Design review of the part built by this model. Coordinates are the model's own, in mm. Face numbers are marked on the shaded views. Coordinates: 2 decimals unless noted, no trailing zeros. Write each loop counter-clockwise with the first axis right and the second up, starting at its lowest first coordinate (ties: lowest second). Pieces come first, ordered by that corner, then holes. Notation, with made-up numbers: (-19, 73.25) -> (10, 73.25) arc R13 ccw to (10, 78.25) -> close; hole circle Ø8 at (65, 65.5). An arc over 180 degrees is marked (long way). Answer in a Markdown table with one row per item. Add a question column.
Item 1: Take a section at A-A, the plane z = 32. Write out the cut boundary in (x, y), and give its area (3 significant figures).
Item 2: To check wall thickness, follow line 1 (X direction, y = 1.35, z = 48); line 2 (X direction, y = 5.5, z = 21.5); line 3 (Y direction, x = -42, z = -11). State the ranges of each line that lie inside material, in increasing order.
Item 3: Take a section at B-B, the plane z = -20. Write out the cut boundary in (x, y).
Item 4: Clearance check with flat-ended pins moving along their axes: P1, Ø1.5, axis at y = 9, z = -24, coming from the +X side; P2, Ø6.5, axis at x = 43.5, z = -16, coming from the +Y side; P3, Ø6, axis at y = 12, z = -2, coming from the -X side. State where each tip first meets the part, or that it passes through.
Item 5: Draft analysis for pull direction X (two halves, no side actions). For the marked faces 1, 2 and 3, state which applies: released by +X, released by -X, zero draft, split by the parting line, or undercut.
Item 6: Take a section at C-C, the plane y = 16.25. Write out the cut boundary in (x, z), and give its area (3 significant figures).
Autodesk Inventor part; units mm, degrees
ref_plane "YZ Plane" through (0, 0, 0) normal (1, 0, 0) x (0, 1, 0)
ref_plane "XZ Plane" through (0, 0, 0) normal (0, 1, 0) x (-1, 0, 0)
ref_plane "XY Plane" through (0, 0, 0) normal (0, 0, 1) x (1, 0, 0)
sketch "Sketch1" plane through (0, 0, 0) normal (0, 1, 0) x (-1, 0, 0)
  line L0 (-47.5, -52) -> (47.5, -52)
  line L1 (47.5, -52) -> (47.5, 52)
  line L2 (47.5, 52) -> (-47.5, 52)
  line L3 (-47.5, 52) -> (-47.5, -52)
  line L4 (-47.5, -52) -> (47.5, 52) construction
  line L5 (47.5, -52) -> (-47.5, 52) construction
  point P0 (0, 0)
  dimension "d0" = 95
  dimension "d1" = 104
extrude "Extrusion1" add sketch "Sketch1" along normal blind 3
sketch "Sketch2" plane through (0, 3, 0) normal (0, 1, 0) x (1, 0, 0)
  line L0 (-47.5, -52) -> (47.5, -52)
  line L1 (37.5, 52) -> (-37.5, 52)
  line L2 (-37.5, 52) -> (-37.5, -52)
  line L3 (-37.5, -52) -> (37.5, -52)
  line L4 (37.5, -52) -> (37.5, 52)
  line L5 (37.5, 52) -> (-37.5, -52) construction
  line L6 (-37.5, 52) -> (37.5, -52) construction
  point P0 (0, 0)
  dimension "d4" = 75
  dimension "d5" = 104
extrude "Extrusion2" add sketch "Sketch2" along normal blind 20
sketch "Sketch3" plane through (0, 0, 0) normal (0, -1, 0) x (1, 0, 0)
  line L0 (-47.5, 52) -> (-43.5, 52)
  line L1 (-43.5, 52) -> (-43.5, 48)
  line L2 (-43.5, 48) -> (-47.5, 48)
  line L3 (-47.5, 48) -> (-47.5, 52)
  line L4 (-47.5, 52) -> (47.5, 52)
  line L5 (47.5, 52) -> (43.5, 52)
  line L6 (43.5, 52) -> (43.5, 48)
  line L7 (43.5, 48) -> (47.5, 48)
  line L8 (47.5, 48) -> (47.5, 52)
  circle A0 centre (-43.5, 48) radius 1.85
  circle A1 centre (-43.5, 32) radius 1.85
  circle A2 centre (-43.5, 16) radius 1.85
  circle A3 centre (-43.5, 0) radius 1.85
  circle A4 centre (-43.5, -16) radius 1.85
  circle A5 centre (-43.5, -32) radius 1.85
  circle A6 centre (-43.5, -48) radius 1.85
  circle A7 centre (43.5, -48) radius 1.85
  circle A8 centre (43.5, -32) radius 1.85
  circle A9 centre (43.5, -16) radius 1.85
  circle A10 centre (43.5, 0) radius 1.85
  circle A11 centre (43.5, 16) radius 1.85
  circle A12 centre (43.5, 32) radius 1.85
  circle A13 centre (43.5, 48) radius 1.85
  point P0 (0, 0)
  dimension "d8" = 4
  dimension "d9" = 4
  dimension "d10" = 4
  dimension "d11" = 4
hole "Hole2" at (-43.5, 0, 48) at (-43.5, 0, 32) at (-43.5, 0, 16) at (-43.5, 0, 0) at (-43.5, 0, -16) at (-43.5, 0, -32) at (-43.5, 0, -48) at (43.5, 0, -48) at (43.5, 0, -32) at (43.5, 0, -16) at (43.5, 0, 0) at (43.5, 0, 16) at (43.5, 0, 32) at (43.5, 0, 48) direction (0, 1, 0) diameter 4 end through all
properties part number "CPD Module"
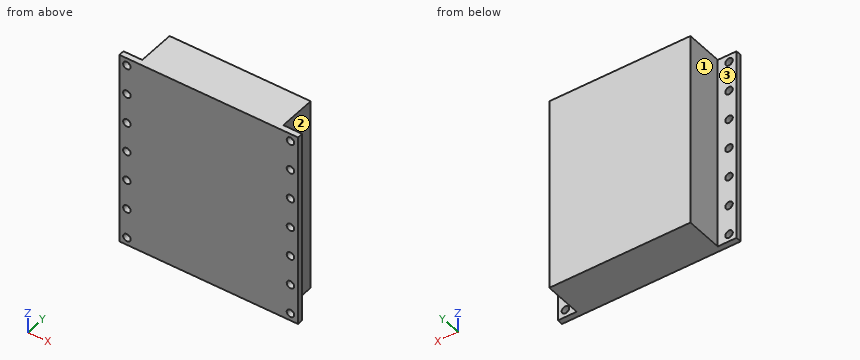
Answers:
| question | item | result |
|---|---|---|
| 1 | outline | (-47.5, 0) -> (-45.5, 0) -> (-45.5, 3) -> (-47.5, 3) -> close; (-41.5, 0) -> (41.5, 0) -> (41.5, 3) -> (37.5, 3) -> (37.5, 23) -> (-37.5, 23) -> (-37.5, 3) -> (-41.5, 3) -> close; (45.5, 0) -> (47.5, 0) -> (47.5, 3) -> (45.5, 3) -> close |
| 1 | area | 1,760 mm^2 |
| 2 | line 1 | x = -47.5 to -45.5, -41.5 to 41.5, 45.5 to 47.5 |
| 2 | line 2 | x = -37.5 to 37.5 |
| 2 | line 3 | y = 0 to 3 |
| 3 | outline | (-47.5, 0) -> (47.5, 0) -> (47.5, 3) -> (37.5, 3) -> (37.5, 23) -> (-37.5, 23) -> (-37.5, 3) -> (-47.5, 3) -> close |
| 4 | P1 | stops at x = 37.5 |
| 4 | P2 | stops at y = 3 |
| 4 | P3 | stops at x = -37.5 |
| 5 | face 1 | released by -X |
| 5 | face 2 | released by +X |
| 5 | face 3 | zero draft |
| 6 | outline | (-37.5, -52) -> (37.5, -52) -> (37.5, 52) -> (-37.5, 52) -> close |
| 6 | area | 7,800 mm^2 |
